```python
from build123d import *

# Parameters (mm, degrees)
F0_W           = 304.8
F0_H           = 41.275
F1_DEPTH       = 4.7625
F3_R           = 4.191
F4_DEPTH       = 4.7635
F5_D           = 3.2639
F5_DEPTH       = 14.605
F5_CSINK_D     = 6.477
F5_CSINK_ANGLE = 82
F5_TIP         = 0.9805744872
F7_DEPTH       = 25.4


with BuildPart() as f1:
    # F0 (on Front) → F1 (new body)
    with BuildSketch(Plane.XZ):
        with Locations((33.2768968371, 36.1280379981)):
            Rectangle(F0_W, F0_H)
    extrude(amount=F1_DEPTH)

    # F3 (on face) → F4 (cut, through all)
    with BuildSketch(Plane(origin=(0, 0, 0), x_dir=(-1, 0, 0), z_dir=(0, 1, 0))):
        with Locations((91.9631031629, 31.9930379981)):
            Circle(F3_R)
        with Locations((-158.5168968371, 31.9930379981)):
            Circle(F3_R)
    extrude(amount=-F4_DEPTH, mode=Mode.SUBTRACT)

    # F5
    with Locations(Plane(origin=(0, 0, 0), x_dir=(-1, 0, 0), z_dir=(0, 1, 0))):
        with Locations((-183.2956468371, 28.1905379981), (-160.2768968371, 54.3842879981), (-33.2768968371, 54.3842879981), (93.7231031629, 54.3842879981), (116.7418531629, 28.1905379981)):
            CounterSinkHole(F5_D / 2, F5_CSINK_D / 2, depth=F5_DEPTH, counter_sink_angle=F5_CSINK_ANGLE)
            with Locations((0, 0, -(F5_DEPTH + F5_TIP / 2))):  # 118° drill point
                Cone(0, F5_D / 2, F5_TIP, mode=Mode.SUBTRACT)

    # F6 (on face) → F7 (cut)
    with BuildSketch(Plane.XZ.offset(4.7625)):
        with BuildLine():
            Line((-38.6665120517, 43.1130379981), (-59.879694274, 43.1130379981))
            ThreePointArc((-59.879694274, 43.1130379981), (-61.9731031629, 36.1280379981), (-59.879694274, 29.1430379981))
            Line((-59.879694274, 29.1430379981), (-38.6665120517, 29.1430379981))
            ThreePointArc((-38.6665120517, 29.1430379981), (-36.5731031629, 36.1280379981), (-38.6665120517, 43.1130379981))
        make_face()
        with BuildLine():
            ThreePointArc((62.9334879483, 29.1430379981), (65.0268968371, 36.1280379981), (62.9334879483, 43.1130379981))
            Line((62.9334879483, 43.1130379981), (41.720305726, 43.1130379981))
            ThreePointArc((41.720305726, 43.1130379981), (39.6268968371, 36.1280379981), (41.720305726, 29.1430379981))
            Line((41.720305726, 29.1430379981), (62.9334879483, 29.1430379981))
        make_face()
    extrude(amount=-F7_DEPTH, mode=Mode.SUBTRACT)


solid = f1.part
```
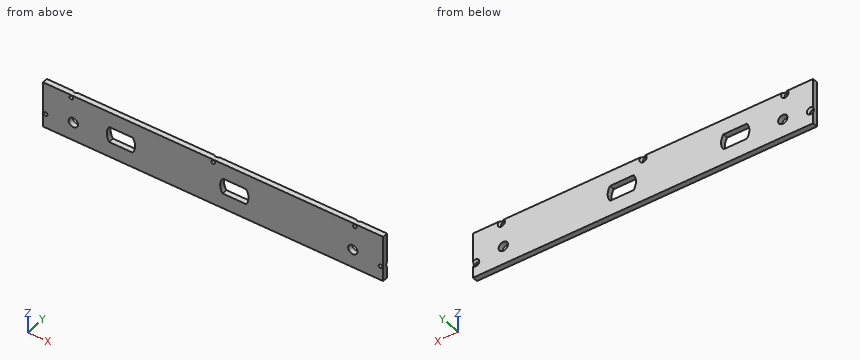
The listing builds one solid part. Answer for the finished solid, in the listing's coordinates (mm). Give positions to 0.01 mm unless a question says otherwise; leave off trailing zeros. Write each loop counter-clockwise with the first axis right and the second up, starting at its lowest first coordinate (ties: lowest second). Pieces come first, ordered by that corner, then holes. Notation, with made-up numbers: M -3.75,-24 L 34.25,-24 A15 ccw 34.25,-17 Z; hole C -24.75,-8.75 d10. An arc over 180 degrees is marked long. Write each question's results on one line, items separated by ' | '.
Q1. Section B-B, the plane y = -2.85 is taken. Count the separate pieces of the cut face and the enclosed holes in it, then the cut area to 3 significant figures.
Output values:
separate pieces: 1 | enclosed holes: 9 | area: 11,800 mm2
Q2. A flat-ended cylindrical pin translates along its axis: P1, Ø5, axis at x = 160.28, z = 54.38, coming from the +Y side. Find the tip coordinate at first contact, or state that the pin passes through.
Output values:
P1: y = -0.84
Q3. Consider L1, parallel to Z at x = 60, y = -1.4; L2, parallel to X at y = -0.9, z = 35; L3, parallel to X at y = -2.9, z = 34. Determine where each line is inside the solid, lowest interval first. Write a range as from..to.
Output values:
L1: 15.49..29.14, 43.11..56.77 | L2: -119.12..-94.88, -89.04..-61.92, -36.62..39.68, 64.98..155.6, 161.44..185.68 | L3: -119.12..-95.64, -88.28..-61.79, -36.75..39.81, 64.85..154.84, 162.2..185.68
Q4. Section A-A, the plane x = -44 is taken. Write down the section's boundary in (y, z).
Output values:
outline: M -4.76,15.49 L 0,15.49 L 0,29.14 L -4.76,29.14 Z; M -4.76,43.11 L 0,43.11 L 0,56.77 L -4.76,56.77 Z
